Source: three-view drawing plus pictorial views. Frame: mm from the lowest corner of the part. Give positions to 0.01 mm unless a question says otherwise; leave off trailing zeros. Order: outer loops, then holes, each group sorted by start corner. A loop starts at its lowest first (then second) coordinate and runs counter-clockwise, first axis right, second up. Notation, with made-up numbers: (-32.75, 2.5) -> (9.25, 2.5) arc R15 cw to (9.25, 24.5) -> close; hole circle Ø7 at (-17.5, 49.25). An arc over 180 degrees is marked (long way). Write item = value, one per line.
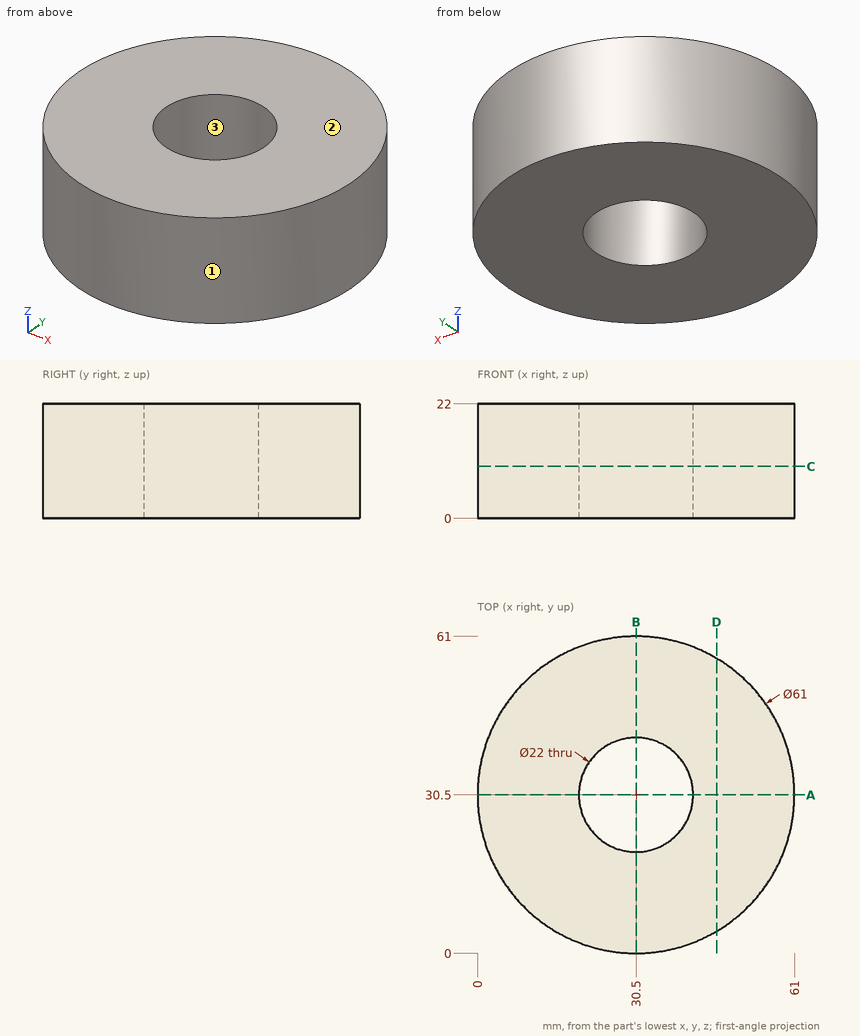
1) Section query D-D (x = 46). Output: boundary loops of the cut face in (y, z), plus the area to 3 significant figures.
Check sheet entries:
outline = (4.23, 0) -> (56.77, 0) -> (56.77, 22) -> (4.23, 22) -> close
area = 1,160 mm²
2) Line query: line 1 (Y direction, x = 30.5, z = 5.5); line 2 (X direction, y = 32.5, z = 16.5); line 3 (X direction, y = 38, z = 16.25). Output: solid intervals per line, ascending. Write a range as from..to.
Check sheet entries:
line_1 = 0..19.5, 41.5..61
line_2 = 0.07..19.68, 41.32..60.93
line_3 = 0.94..22.45, 38.55..60.06
3) Section query A-A (y = 30.5). Output: boundary loops of the cut face in (x, z).
Check sheet entries:
outline = (0, 0) -> (19.5, 0) -> (19.5, 22) -> (0, 22) -> close; (41.5, 0) -> (61, 0) -> (61, 22) -> (41.5, 22) -> close
4) Section query C-C (z = 10). Output: boundary loops of the cut face in (x, y).
Check sheet entries:
outline = circle Ø61 at (30.5, 30.5); hole circle Ø22 at (30.5, 30.5)
5) Mould query, pull axis Y, two halves, no side actions, for the marked faces 1, 2 and 3. Classes: +Y half, -Y half, draft (parallel to the pull), parting line (faces both ways), or undercut.
Check sheet entries:
face_1 = parting line
face_2 = draft
face_3 = undercut
6) First-contact query: P1, Ø10, axis at x = 47.5, z = 10.5, coming from the +Y side; P2, Ø13, axis at x = 30.5, y = 30.5, coming from the -Z side; P3, Ø6, axis at x = 38, z = 12, coming from the +Y side; P4, Ø3, axis at y = 36, z = 6, coming from the -X side. Flat tips, straight axial feed; report the tip coordinate or a pass-through.
Check sheet entries:
P1 = 58.54
P2 = through
P3 = 60.67
P4 = 0.26
